Verification items for the finished model (mm, model axes). Give positions to 0.01 mm unless a question says otherwise; leave off trailing zeros. Order: outer loops, then holes, each group sorted by start corner. A loop starts at its lowest first (then second) coordinate and runs counter-clockwise, first axis right, second up. Notation, with made-up numbers: (9.25, -6) - (32.25, -6) arc R11 cw to (32.25, 8) - close; hole circle Ø2 at (24, 6). An arc over 180 degrees is marked (long way). Answer as a JSON object with one key per item and string values. Group by question number.
(1) Section check C-C (z = 3.2). Record the boundary of the cut face in (x, y).
(2) Depth check by flat-ended pin: pin 1 Ø1.7 at (y, z) = (1, -1.5) entering from -X; pin 2 Ø0.5 at (x, y) = (-4.5, 0) entering from +Z; pin 3 Ø0.5 at (x, y) = (-5, 0) entering from -Z. Enter the tip coordinate at first touch or a pass-through.
(3) Section check B-B (x = -2.25). Record the boundary of the cut face in (y, z).
(4) Section check A-A (y = -0.6). Record the boundary of the cut face in (x, z) (3 decimals).
(5) Thickness scan on line 1 (Z direction, x = -1.65, y = -0.3); line 2 (X direction, y = 1.35, z = -1.75); line 3 (Y direction, x = -4, z = 5). Record the ranges inside material, lowest first.
(6) Section check D-D (x = -4.75). Record the boundary of the cut face in (y, z).
```python
from build123d import *

# Parameters (mm, degrees)
F0_W     = 6.7
F0_H     = 12.8
F0_R     = 1
F1_DEPTH = 2.85
F2_W     = 0.6
F2_H     = 0.6
F3_DEPTH = 3.4
F4_W     = 3
F4_H     = 1.25
F5_DEPTH = 0.6


with BuildPart() as f1:
    # F0 (on Front) → F1 (new body, symmetric)
    with BuildSketch(Plane.XZ):
        Rectangle(F0_W, F0_H)
        with Locations((-1.65, -3.2)):
            Circle(F0_R, mode=Mode.SUBTRACT)
        with Locations((-1.65, 3.2)):
            Circle(F0_R, mode=Mode.SUBTRACT)
    extrude(amount=F1_DEPTH, both=True)

    # F2 (on face) → F3 (join)
    with BuildSketch(Plane(origin=(-3.35, 0, 0), x_dir=(0, -1, 0), z_dir=(-1, 0, 0))):
        Rectangle(F2_W, F2_H)
        with Locations((0, 5)):
            Rectangle(F2_W, F2_H)
        with Locations((0, -5)):
            Rectangle(F2_W, F2_H)
    extrude(amount=F3_DEPTH)

    # F4 (on face) → F5 (join)
    with BuildSketch(Plane.YZ.offset(3.35)):
        with Locations((0, 1.9)):
            Rectangle(F4_W, F4_H)
    extrude(amount=F5_DEPTH)


solid = f1.part
```
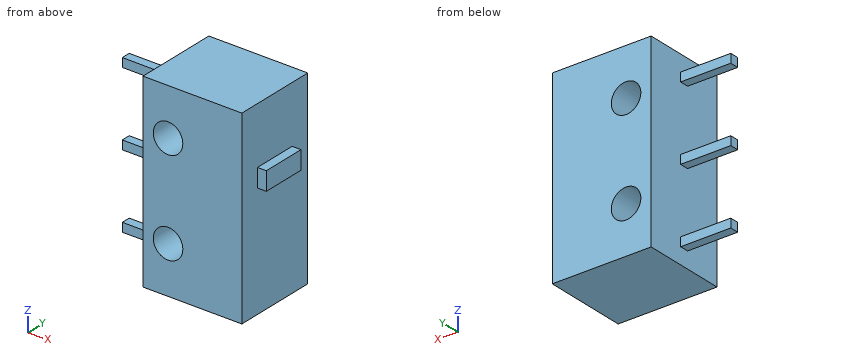
Solutions:
{
 "1": {"outline": "(-3.35, -2.85) - (-2.65, -2.85) - (-2.65, 2.85) - (-3.35, 2.85) - close; (-0.65, -2.85) - (3.35, -2.85) - (3.35, 2.85) - (-0.65, 2.85) - close"},
 "2": {"pin 1": "stops at x = -3.35", "pin 2": "stops at z = 5.3", "pin 3": "stops at z = -5.3"},
 "3": {"outline": "(-2.85, -6.4) - (2.85, -6.4) - (2.85, -4) - (-2.85, -4) - close; (-2.85, -2.4) - (2.85, -2.4) - (2.85, 2.4) - (-2.85, 2.4) - close; (-2.85, 4) - (2.85, 4) - (2.85, 6.4) - (-2.85, 6.4) - close"},
 "4": {"outline": "(-3.35, -6.4) - (3.35, -6.4) - (3.35, 1.275) - (3.95, 1.275) - (3.95, 2.525) - (3.35, 2.525) - (3.35, 6.4) - (-3.35, 6.4) - close; hole circle Ø2 at (-1.65, -3.2); hole circle Ø2 at (-1.65, 3.2)"},
 "5": {"line 1": "z = -6.4 to -4.2, -2.2 to 2.2, 4.2 to 6.4", "line 2": "x = -3.35 to 3.35", "line 3": "y = -0.3 to 0.3"},
 "6": {"outline": "(-0.3, -5.3) - (0.3, -5.3) - (0.3, -4.7) - (-0.3, -4.7) - close; (-0.3, -0.3) - (0.3, -0.3) - (0.3, 0.3) - (-0.3, 0.3) - close; (-0.3, 4.7) - (0.3, 4.7) - (0.3, 5.3) - (-0.3, 5.3) - close"}
}
